Autodesk Inventor part; units mm, degrees
ref_plane "YZ Plane" through (0, 0, 0) normal (1, 0, 0) x (0, 1, 0)
ref_plane "XZ Plane" through (0, 0, 0) normal (0, 1, 0) x (-1, 0, 0)
ref_plane "XY Plane" through (0, 0, 0) normal (0, 0, 1) x (1, 0, 0)
sketch "Sketch1" plane through (0, 0, 0) normal (0, 1, 0) x (-1, 0, 0)
  circle A0 centre (0, 0) radius 20.0025
  line L0 (-11.6713, 11.6713) -> (11.6713, 11.6713)
  line L1 (11.6713, 11.6713) -> (11.6713, -11.6713)
  line L2 (11.6713, -11.6713) -> (-11.6713, -11.6713)
  line L3 (-11.6713, -11.6713) -> (-11.6713, 11.6713)
  line L4 (-11.6713, 11.6713) -> (11.6713, -11.6713) construction
  line L5 (11.6713, 11.6713) -> (-11.6713, -11.6713) construction
  circle A1 centre (11.6713, -11.6713) radius 1.2446
  circle A2 centre (-11.6713, -11.6713) radius 1.2446
  circle A3 centre (-11.6713, 11.6713) radius 1.2446
  circle A4 centre (11.6713, 11.6713) radius 1.2446
  dimension "d0" = 40.005
  dimension "d1" = 23.3426
  dimension "d2" = 23.3426
  dimension "d3" = 2.4892
  dimension "d4" = 2.4892
  dimension "d5" = 2.4892
  dimension "d6" = 2.4892
extrude "Extrusion1" add sketch "Sketch1" along normal blind 3.81 contours A0 | L0 A4 L1 A1 L2 A2 L3 A3
sketch "Sketch3" plane through (0, 0, 0) normal (0, -1, 0) x (1, 0, 0)
  circle A0 centre (0, 0) radius 1.5875
  dimension "d10" = 3.175
extrude "Extrusion2" cut sketch "Sketch3" against normal blind 6.35
sketch "Sketch5" plane through (0, 3.81, 0) normal (0, 1, 0) x (1, 0, 0)
  circle A0 centre (0, 0) radius 20.0025
sketch "Sketch6" plane through (0, 3.81, 0) normal (0, 1, 0) x (1, 0, 0)
  line L0 (-11.6713, 11.6713) -> (11.6713, 11.6713)
  line L1 (11.6713, 11.6713) -> (11.6713, -11.6713)
  line L2 (11.6713, -11.6713) -> (-11.6713, -11.6713)
  line L3 (-11.6713, -11.6713) -> (-11.6713, 11.6713)
  circle A0 centre (0, 0) radius 1.5875
  line L4 (-11.6713, 11.6713) -> (11.6713, -11.6713) construction
  line L5 (11.6713, 11.6713) -> (-11.6713, -11.6713) construction
  circle A1 centre (-11.6713, 11.6713) radius 3.175
  circle A2 centre (11.6713, 11.6713) radius 3.175
  circle A3 centre (11.6713, -11.6713) radius 3.175
  circle A4 centre (-11.6713, -11.6713) radius 1.2446
  circle A5 centre (-11.6713, -11.6713) radius 3.175
  dimension "d13" = 23.3426
  dimension "d14" = 6.35
  dimension "d15" = 6.35
  dimension "d16" = 6.35
  dimension "d17" = 6.35
extrude "Extrusion3" add sketch "Sketch5" along normal blind 6.35
sketch "Sketch7" plane through (0, 10.16, 0) normal (0, 1, 0) x (1, 0, 0)
  line L0 (-11.6713, -11.6713) -> (11.6713, -11.6713)
  line L1 (11.6713, -11.6713) -> (11.6713, 11.6713)
  line L2 (11.6713, 11.6713) -> (-11.6713, 11.6713)
  line L3 (-11.6713, 11.6713) -> (-11.6713, -11.6713)
  circle A0 centre (0, 0) radius 1.5875
  line L4 (-11.6713, -11.6713) -> (11.6713, 11.6713) construction
  line L5 (11.6713, -11.6713) -> (-11.6713, 11.6713) construction
  circle A1 centre (-11.6713, 11.6713) radius 1.2446
  circle A2 centre (-11.6713, 11.6713) radius 2.54
  circle A3 centre (11.6713, 11.6713) radius 1.2446
  circle A4 centre (11.6713, 11.6713) radius 2.54
  circle A5 centre (11.6713, -11.6713) radius 1.2446
  circle A6 centre (11.6713, -11.6713) radius 2.54
  circle A7 centre (-11.6713, -11.6713) radius 1.2446
  circle A8 centre (-11.6713, -11.6713) radius 2.54
  dimension "d20" = 23.3426
  dimension "d21" = 23.3426
  dimension "d22" = 5.08
  dimension "d23" = 5.08
  dimension "d24" = 5.08
  dimension "d25" = 5.08
extrude "Extrusion4" cut sketch "Sketch7" against normal blind 6.35 contours L3 A7 L0 | L0 A7 L3 | A7 L3 A8 L0 | L0 A8 L3 A7 | A6 L1 A5 L0 | L0 A5 L1 A6 | A2 L2 A1 L3 | L3 A1 L2 A2 | A5 L1 L0 | L0 L1 A5 | A1 L2 L3 | L3 L2 A1 | A4 L2 A3 L1 | L1 A3 L2 A4 | A3 L2 L1 | L1 L2 A3
properties part number "CO-0-01-Planetary1"
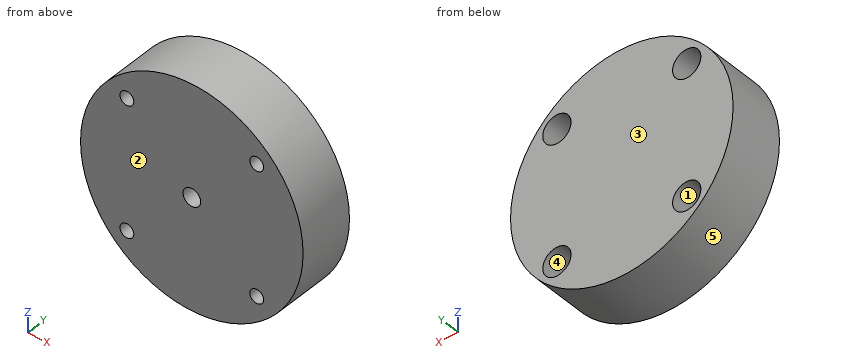
Design review of the part built by this model. Coordinates are the model's own, in mm. Face numbers are marked on the shaded views. A direction names the side the tool comes from. Coordinates: 2 decimals unless noted, no trailing zeros. Order: outer loops, then holes, each group sorted by start corner. A loop starts at its lowest first (then second) coordinate and runs counter-clockwise, first axis right, second up. Notation, with made-up numbers: (17.5, 54.25) -> (70.5, 54.25) arc R8 ccw to (70.5, 65.25) -> close; hole circle Ø9 at (-10, -22.5). An arc over 180 degrees is marked (long way). One line per item, written item: value. Start each with the question number.
Q1. Insertion check: pin 1 Ø1 at (x, y) = (15.5, 2.5) entering from -Z; pin 2 Ø2.5 at (x, z) = (12.5, -12.5) entering from +Y; pin 3 Ø1 at (y, z) = (2, -14.5) entering from -X. Each pin has a flat end and moves straight along its axis. Give the tip position at first contact, or say it passes through.
Q2. Take a section at C-C, the plane y = 4.75. State the section outline as (x, z) points (1 decimal), then the cut area to 3 significant figures.
Q3. For probe 1 along Z at (x, y) = (-13, 5); probe 2 along X at (y, z) = (1, -11); probe 3 along X at (y, z) = (0.5, 0.5), list the stretches that pass through material, from the lowest coordinate up.
Q4. Take a section at A-A, the plane z = 0. State the section outline as (x, y) points.
Q5. Take a section at B-B, the plane x = 0. State the section outline as (y, z) points, then the cut area to 3 significant figures.
Q6. Tool access review of the marked faces 1 and 2: name each direction out of +Z, -Z, +X, -X, +Y, -Y from which nothing blocks a thin tool from reaching the whole face with its end or side.
Q7. Take a section at D-D, the plane z = -11. State the section outline as (x, y) points.
Q8. Mouldability with a two-part tool opening along X and no side actions: class the marked faces 3, 4 and 5 as pulls with the +X half, pulls with the -X half, needs draft (parallel to the pull), parting line crosses it, or undercut.
Values follow:
1. pin 1: stops at z = -13.23
1. pin 2: stops at y = 3.81
1. pin 3: stops at x = -14.29
2. outline: circle Ø40 at (0, 0); hole circle Ø5.1 at (-11.7, -11.7); hole circle Ø5.1 at (-11.7, 11.7); hole circle Ø5.1 at (11.7, -11.7); hole circle Ø5.1 at (11.7, 11.7)
2. area: 1,180 mm2
3. probe 1: z = -15.2 to -13.84, -9.51 to 9.51, 13.84 to 15.2
3. probe 2: x = -16.71 to -12.72, -10.62 to 10.62, 12.72 to 16.71
3. probe 3: x = -20 to -1.51, 1.51 to 20
4. outline: (-20, 0) -> (-1.59, 0) -> (-1.59, 3.81) -> (1.59, 3.81) -> (1.59, 0) -> (20, 0) -> (20, 10.16) -> (-20, 10.16) -> close
5. outline: (0, -20) -> (10.16, -20) -> (10.16, 20) -> (0, 20) -> (0, 1.59) -> (3.81, 1.59) -> (3.81, -1.59) -> (0, -1.59) -> close
5. area: 394 mm2
6. face 1: +Y
6. face 2: +Z, -Z, +X, -X, -Y
7. outline: (-16.71, 0) -> (-12.72, 0) -> (-12.72, 3.81) -> (-14.12, 3.81) -> (-14.12, 10.16) -> (-16.71, 10.16) -> close; (-10.62, 0) -> (10.62, 0) -> (10.62, 3.81) -> (9.22, 3.81) -> (9.22, 10.16) -> (-9.22, 10.16) -> (-9.22, 3.81) -> (-10.62, 3.81) -> close; (12.72, 0) -> (16.71, 0) -> (16.71, 10.16) -> (14.12, 10.16) -> (14.12, 3.81) -> (12.72, 3.81) -> close
8. face 3: needs draft
8. face 4: undercut
8. face 5: parting line crosses it
